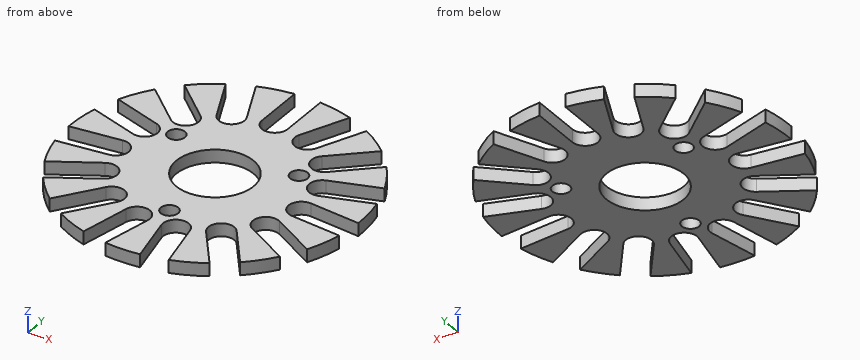
```python
from build123d import *

# Parameters (mm, degrees)
SKETCH1_R           = 1.35
SKETCH1_R_2         = 6
BOSS_EXTRUDE1_DEPTH = 2


with BuildPart() as part:
    # Sketch1 → Boss-Extrude1 (new body)
    with BuildSketch(Plane(origin=(0, 0, 0), x_dir=(-1, 0, 0), z_dir=(0, 0, -1))):
        with BuildLine():
            Line((-15.316309042, 17.102154929), (-9.437338757, 11.808706309))
            ThreePointArc((-9.437338757, 11.808706309), (-9.289310319, 8.984155445), (-12.113861182, 8.836127007))
            Line((-12.113861182, 8.836127007), (-17.992831467, 14.129575627))
            ThreePointArc((-17.992831467, 14.129575627), (-19.485571585, 11.870022867), (-20.696031618, 9.447495623))
            Line((-20.696031618, 9.447495623), (-13.172285497, 7.002882316))
            ThreePointArc((-13.172285497, 7.002882316), (-11.888206454, 4.482735294), (-14.408353475, 3.198656251))
            Line((-14.408353475, 3.198656251), (-21.932099596, 5.643269556))
            ThreePointArc((-21.932099596, 5.643269556), (-22.376742646, 2.971913289), (-22.497222312, 0.266486078))
            Line((-22.497222312, 0.266486078), (-14.62962441, 1.093403939))
            ThreePointArc((-14.62962441, 1.093403939), (-12.431523692, -0.686582926), (-14.211510557, -2.884683643))
            Line((-14.211510557, -2.884683643), (-22.079108459, -3.711601503))
            ThreePointArc((-22.079108459, -3.711601503), (-21.398771617, -6.332859507), (-20.408438887, -8.853393742))
            Line((-20.408438887, -8.853393742), (-13.557368355, -4.897926326))
            ThreePointArc((-13.557368355, -4.897926326), (-10.825317547, -5.629977134), (-11.557368355, -8.362027942))
            Line((-11.557368355, -8.362027942), (-18.408438886, -12.317495358))
            ThreePointArc((-18.408438886, -12.317495358), (-16.720758571, -14.435415779), (-14.790850969, -16.335233771))
            Line((-14.790850969, -16.335233771), (-10.140920148, -9.935153049))
            ThreePointArc((-10.140920148, -9.935153049), (-7.347315654, -9.492689564), (-6.90485217, -12.286294058))
            Line((-6.90485217, -12.286294058), (-11.554782995, -18.686374777))
            ThreePointArc((-11.554782995, -18.686374777), (-9.151574469, -19.934749931), (-6.615790555, -20.885355888))
            Line((-6.615790555, -20.885355888), (-4.971014718, -13.147293963))
            ThreePointArc((-4.971014718, -13.147293963), (-2.598896135, -11.606822144), (-1.058424316, -13.978940727))
            Line((-1.058424316, -13.978940727), (-2.703200152, -21.717002651))
            ThreePointArc((-2.703200152, -21.717002651), (-3e-09, -21.879977134), (2.703200146, -21.717002651))
            Line((2.703200146, -21.717002651), (1.058424314, -13.978940725))
            ThreePointArc((1.058424314, -13.978940725), (2.598896135, -11.606822143), (4.971014718, -13.147293963))
            Line((4.971014718, -13.147293963), (6.615790554, -20.885355888))
            ThreePointArc((6.615790554, -20.885355888), (9.151574469, -19.934749931), (11.554782995, -18.686374777))
            Line((11.554782995, -18.686374777), (6.904852169, -12.286294058))
            ThreePointArc((6.904852169, -12.286294058), (7.347315653, -9.492689564), (10.140920146, -9.935153048))
            Line((10.140920146, -9.935153048), (14.790850972, -16.335233768))
            ThreePointArc((14.790850972, -16.335233768), (16.720758571, -14.435415779), (18.408438883, -12.317495361))
            Line((18.408438883, -12.317495361), (11.557368352, -8.362027946))
            ThreePointArc((11.557368352, -8.362027946), (10.825317543, -5.629977135), (13.557368354, -4.897926327))
            Line((13.557368354, -4.897926327), (20.408438886, -8.853393742))
            ThreePointArc((20.408438886, -8.853393742), (21.398771616, -6.332859507), (22.079108458, -3.711601502))
            Line((22.079108458, -3.711601502), (14.211510556, -2.884683643))
            ThreePointArc((14.211510556, -2.884683643), (12.431523691, -0.686582926), (14.629624409, 1.093403939))
            Line((14.629624409, 1.093403939), (22.497222311, 0.266486078))
            ThreePointArc((22.497222311, 0.266486078), (22.376742645, 2.971913287), (21.932099596, 5.643269552))
            Line((21.932099596, 5.643269552), (14.408353473, 3.19865625))
            ThreePointArc((14.408353473, 3.19865625), (11.888206452, 4.482735295), (13.172285497, 7.002882316))
            Line((13.172285497, 7.002882316), (20.696031618, 9.447495621))
            ThreePointArc((20.696031618, 9.447495621), (19.485571584, 11.870022866), (17.992831465, 14.129575628))
            Line((17.992831465, 14.129575628), (12.113861182, 8.836127007))
            ThreePointArc((12.113861182, 8.836127007), (9.289310318, 8.984155445), (9.437338756, 11.808706308))
            Line((9.437338756, 11.808706308), (15.316309041, 17.102154929))
            ThreePointArc((15.316309041, 17.102154929), (13.225168178, 18.822905238), (10.94243932, 20.279957294))
            Line((10.94243932, 20.279957294), (7.724772239, 13.052958714))
            ThreePointArc((7.724772239, 13.052958714), (5.084208037, 12.039341086), (4.070590408, 14.679905287))
            Line((4.070590408, 14.679905287), (7.288257486, 21.906903868))
            ThreePointArc((7.288257486, 21.906903868), (4.67801304, 22.628343883), (1.999999993, 23.030957697))
            Line((1.999999993, 23.030957697), (1.999999993, 15.120022866))
            ThreePointArc((1.999999993, 15.120022866), (-1e-09, 13.120022872), (-1.999999995, 15.120022866))
            Line((-1.999999995, 15.120022866), (-1.999999995, 23.030957697))
            ThreePointArc((-1.999999995, 23.030957697), (-4.67801304, 22.628343883), (-7.288257483, 21.906903869))
            Line((-7.288257483, 21.906903869), (-4.070590409, 14.679905287))
            ThreePointArc((-4.070590409, 14.679905287), (-5.084208039, 12.039341085), (-7.72477224, 13.052958715))
            Line((-7.72477224, 13.052958715), (-10.942439317, 20.279957296))
            ThreePointArc((-10.942439317, 20.279957296), (-13.225168177, 18.822905239), (-15.316309042, 17.102154929))
        make_face()
        with Locations((9.526279442, 6.120022866)):
            Circle(SKETCH1_R, mode=Mode.SUBTRACT)
        with Locations((-9.526279442, 6.120022866)):
            Circle(SKETCH1_R, mode=Mode.SUBTRACT)
        with Locations((0, -10.379977134)):
            Circle(SKETCH1_R, mode=Mode.SUBTRACT)
        with Locations((0, 0.620022866)):
            Circle(SKETCH1_R_2, mode=Mode.SUBTRACT)
    extrude(amount=-BOSS_EXTRUDE1_DEPTH)


solid = part.part
```
Geometry: final body of the model. Coordinates: model frame, mm. Coordinates: 2 decimals unless noted, no trailing zeros. Order: outer loops, then holes, each group sorted by start corner. A loop starts at its lowest first (then second) coordinate and runs counter-clockwise, first axis right, second up. Notation, with made-up numbers: (49.25, 62) - (94.25, 62) arc R9 cw to (94.25, 79) - close; hole circle Ø1 at (86, -21.5). An arc over 180 degrees is marked (long way). Return JSON: item names as keys, results as strings. Group by question number.
1. Cut plane D-D (z = 1.2). Count the separate pieces of the cut face and the enclosed holes in it, plus the area to 3 significant figures.
2. Material intervals for line 1 along Y through (x, z) = (0, 1); line 2 along Y through (x, z) = (-18.5, 1); line 3 along X through (y, z) = (13, 1), sorted ascending. Write a range as [from, to].
3. Cut plane C-C (x = 16.5). Output: boundary loops of the cut face in (y, z), plus the area to 3 significant figures.
4. Pin query (flat end, axial travel): pin 1 (1 mm diameter, centred on y = 10.5, z = 1, fed in from -X); pin 2 (1 mm diameter, centred on y = 19.5, z = 1, fed in from +X). Return the tip coordinate at first contact, or that it passes through.
5. Cut plane B-B (y = 18). Output: boundary loops of the cut face in (x, z).
6. Cut plane A-A (x = 0). Output: boundary loops of the cut face in (y, z).
Resolved:
{
 "1": {"separate pieces": "1", "enclosed holes": "4", "area": "888 mm²"},
 "2": {"line 1": "y = [-21.88, -11.73], [-9.03, -5.38], [6.62, 13.12]", "line 2": "y = [-7.75, -3.34], [0.69, 4.53], [8.73, 13.43]", "line 3": "x = [-18.79, -16.74], [-10.76, -7.7], [-4.1, 4.1], [7.7, 10.76], [16.74, 18.79]"},
 "3": {"outline": "(-14.68, 0) - (-11.22, 0) - (-11.22, 2) - (-14.68, 2) - close; (-6.6, 0) - (-3.13, 0) - (-3.13, 2) - (-6.6, 2) - close; (0.9, 0) - (3.88, 0) - (3.88, 2) - (0.9, 2) - close; (8.08, 0) - (12.79, 0) - (12.79, 2) - (8.08, 2) - close", "area": "29.2 mm²"},
 "4": {"pin 1": "stops at x = -20.45", "pin 2": "stops at x = 12.98"},
 "5": {"outline": "(-14.29, 0) - (-9.93, 0) - (-9.93, 2) - (-14.29, 2) - close; (-5.55, 0) - (-2, 0) - (-2, 2) - (-5.55, 2) - close; (2, 0) - (5.55, 0) - (5.55, 2) - (2, 2) - close; (9.93, 0) - (14.29, 0) - (14.29, 2) - (9.93, 2) - close"},
 "6": {"outline": "(-21.88, 0) - (-11.73, 0) - (-11.73, 2) - (-21.88, 2) - close; (-9.03, 0) - (-5.38, 0) - (-5.38, 2) - (-9.03, 2) - close; (6.62, 0) - (13.12, 0) - (13.12, 2) - (6.62, 2) - close"}
}
